Autodesk Inventor part; units mm, degrees
ref_plane "Work Plane3" through (0, 1.2, 0) normal (0, 1, 0) x (1, 0, 0)
ref_plane "YZ Plane" through (0, 0, 0) normal (1, 0, 0) x (0, 1, 0)
ref_plane "XZ Plane" through (0, 0, 0) normal (0, 1, 0) x (-1, 0, 0)
sketch "Sketch1" plane through (0, 0, 0) normal (0, 1, 0) x (-1, 0, 0)
  circle A0 centre (0, 0) radius 1.1
  arc A1 (3.1, 0) -> (-3.1, 0) centre (0, 0) ccw
  circle A2 centre (0, -58) radius 1.1
  arc A3 (-3.1, -58) -> (3.1, -58) centre (0, -58) ccw
  line L0 (3.1, -58) -> (3.1, -54.5)
  line L1 (-3.1, -58) -> (-3.1, -54.5)
  line L2 (3.1, -54.5) -> (-3.1, -54.5)
  line L3 (3.1, -3.5) -> (-3.1, -3.5)
  line L4 (-3.1, -3.5) -> (-3.1, 0)
  line L5 (3.1, 0) -> (3.1, -3.5)
  line L6 (3.1, -55.5) -> (-3.1, -55.5)
  line L7 (3.1, -2.5) -> (-3.1, -2.5)
  line L8 (-0.1, -2.5) -> (-0.1, -3.5)
  dimension "d0" = 2.2
  dimension "d1" = 2
  dimension "d2" = 2.2
  dimension "d3" = 2
  dimension "d4" = 58
  dimension "d5" = 3.5
  dimension "d6" = 3.5
  dimension "d7" = 1
  dimension "d8" = 1
  dimension "d17" = 0.1
extrude "Extrusion1" add sketch "Sketch1" along normal blind 2 contours L1 L6 L0 A3
extrude "Extrusion5" add sketch "Sketch1" along normal blind 1 contours L5 L7 L4 A1 | L5 L3 L8 L7
extrude "Extrusion2" add sketch "Sketch1" along normal blind 16.6 contours L7 L8 L3 L4 | L1 L2 L0 L6
sketch "Sketch2" plane through (0, 16.6, 0) normal (0, 1, 0) x (1, 0, 0)
  line L0 (-3.1, 2.5) -> (-3.1, 0) construction
  line L1 (3.1, 55.5) -> (3.1, 58) construction
  line L2 (-3.1, 2.5) -> (3.1, 2.5)
  line L3 (3.1, 2.5) -> (3.1, 55.5)
  line L4 (3.1, 55.5) -> (-3.1, 55.5)
  line L5 (-3.1, 55.5) -> (-3.1, 2.5)
  line L6 (3.1, 3.5) -> (0.1, 3.5) construction
  line L7 (-3.1, 54.5) -> (3.1, 54.5) construction
  line L8 (-1.7, 3.5) -> (1.7, 3.5)
  line L9 (1.7, 3.5) -> (1.7, 54.5)
  line L10 (1.7, 54.5) -> (-1.7, 54.5)
  line L11 (-1.7, 54.5) -> (-1.7, 3.5)
  line L12 (3.1, 3.5) -> (-3.1, 3.5)
  line L13 (-0.1, 3.5) -> (-0.1, 2.5)
  line L14 (0.1, 3.5) -> (0.1, 2.5)
  point P0 (0, 0)
  point P1 (0, 3.5)
  dimension "d13" = 1.4
  dimension "d14" = 1.4
  dimension "d37" = 0.2
  dimension "d38" = 0.1
extrude "Extrusion3" add sketch "Sketch2" along normal blind 2 contours L5 L12 L8 L13 L2 | L5 L4 L3 L12 L9 L10 L11 | L14 L8 L12 L3 L2
ref_plane "Work Plane3" through (0, 1.2, 0) normal (0, 1, 0) x (1, 0, 0)
sketch "Sketch4" plane through (0, 1.2, 0) normal (0, 1, 0) x (1, 0, 0)
  arc A0 (-3.1, 0) -> (3.1, 0) centre (0, 0) ccw
  circle A1 centre (0, 0) radius 1.1
  line L0 (-3.1, 3.5) -> (-3.1, 0) construction
  line L1 (3.1, 0) -> (3.1, 3.5) construction
  line L2 (3.1, 2.3) -> (3.1, 0)
  line L3 (3.1, 2.5) -> (0.1, 2.5) construction
  line L4 (-0.1, 2.3) -> (-0.1, 3.5)
  line L5 (-0.1, 3.5) -> (-3.1, 3.5)
  line L6 (3.1, 2.5) -> (0.1, 2.5)
  line L7 (-3.1, 2.5) -> (-0.1, 2.5)
  line L8 (-0.1, 2.3) -> (3.1, 2.3)
  line L9 (-3.1, 0) -> (-3.1, 3.5)
  dimension "d28" = 0.1
  dimension "d29" = 1
  dimension "d30" = 0.2
extrude "Extrusion6" add sketch "Sketch4" along normal blind 1
extrude "Extrusion8" add sketch "Sketch4" along normal up to surface (15.4 mm away) contours L9 L5 L4 L7
equation "\"d0\" = bolt_thread_diameter + 2 * tol"
equation "\"d1\" = thickness"
equation "\"d2\" = bolt_thread_diameter + 2 * tol"
equation "\"d3\" = thickness"
equation "\"d5\" = hole_pin_separation - tol"
equation "\"d6\" = hole_pin_separation - tol"
equation "\"d7\" = minor_thickness"
equation "\"d8\" = minor_thickness"
equation "\"d9\" = thickness"
equation "\"d24\" = 0.5 * thickness"
equation "\"d11\" = wire_height + pin_base_height + tol"
equation "\"d13\" = overhang"
equation "\"d14\" = overhang"
equation "\"d37\" = 2 * tol"
equation "\"d15\" = thickness"
equation "\"d29\" = minor_thickness"
equation "\"d30\" = 2 * tol"
equation "\"d31\" = 0.5 * thickness"
equation "\"d35\" = 0.5 * thickness"
equation "\"wire_height\" = 14"
equation "\"hole_separation\" = 58"
equation "\"pin_base_height\" = 2.5"
equation "\"hole_pin_separation\" = 3.6"
equation "\"minor_thickness\" = 1"
equation "\"overhang\" = 1.4"
equation "\"d26\" = 2 * tol"
properties part number "WIRE_HOUSING" material "PC/ABS Plastic"
Verification items for the finished model (mm, model axes). A direction names the side the tool comes from. Round coordinates to 2 decimals unless told otherwise and drop trailing zeros. Order: outer loops, then holes, each group sorted by start corner. A loop starts at its lowest first (then second) coordinate and runs counter-clockwise, first axis right, second up. Notation, with made-up numbers: (43, -32) -> (90, -32) arc R11 ccw to (90, -14) -> close; hole circle Ø11 at (54, -38.75). An arc over 180 degrees is marked (long way). Put each result on its own line as item: value.
1) Section check B-B (z = -37). Record the cut outline in (x, y).
Final values:
outline: (-3.1, 16.6) -> (-1.7, 16.6) -> (-1.7, 18.6) -> (-3.1, 18.6) -> close; (1.7, 16.6) -> (3.1, 16.6) -> (3.1, 18.6) -> (1.7, 18.6) -> close
2) Set-up check for faces 4 (the flat face through (0, 10, -55.5)), 5 (the flat face through (2, 16.6, -29)), 6 (the flat face through (1.7, 18, -29)): record each of +Z, -Z, +X, -X, +Y, -Y from which the full face is reachable in a straight line by a thin tool's end or side.
Final values:
face 4: -Z, +X, -X, +Y
face 5: +X, -X, -Y
face 6: +Y, -Y
3) Depth check by flat-ended pin: pin 1 (3 mm diameter, centred on x = -2, z = -18, fed in from -Y); pin 2 (1.8 mm diameter, centred on x = 0, z = -58, fed in from -Y); pin 3 (1.9 mm diameter, centred on x = -1.5, z = 1, fed in from +Y); pin 4 (3 mm diameter, centred on x = -1, z = 1, fed in from -Y). Enter the tip coordinate at first touch or a pass-through.
Final values:
pin 1: stops at y = 16.6
pin 2: passes through
pin 3: stops at y = 2.2
pin 4: stops at y = 0
4) Material ranges on line 1 (Z direction, x = 0, y = 0.5); line 2 (Z direction, x = 0, y = 1.75); line 3 (X direction, y = 1.7, z = 0), recorded low to high.
Final values:
line 1: z = -61.1 to -59.1, -56.9 to -54.5, -3.5 to -1.1, 1.1 to 3.1
line 2: z = -61.1 to -59.1, -56.9 to -54.5, -2.3 to -1.1, 1.1 to 3.1
line 3: x = -3.1 to -1.1, 1.1 to 3.1
5) Mould release check, pull along X, two halves, no side actions. Record for faces 1 (the flat face through (-3.1, 17, -29)), 2 (the flat face through (-2, 10, -2.5)), 3 (the cylindrical face through (-1.05, 0.49, -0.33)): +X half, -X half, draft (parallel to the pull), parting line (faces both ways), or undercut.
Final values:
face 1: -X half
face 2: draft
face 3: undercut
6) Section check A-A (y = 12.25). Record the cut outline in (x, z).
Final values:
outline: (-3.1, -55.5) -> (3.1, -55.5) -> (3.1, -54.5) -> (-3.1, -54.5) -> close; (-3.1, -3.5) -> (-0.1, -3.5) -> (-0.1, -2.5) -> (-3.1, -2.5) -> close; (0.1, -3.5) -> (3.1, -3.5) -> (3.1, -2.5) -> (0.1, -2.5) -> close
7) Section check C-C (x = 2.5). Record the cut outline in (y, z).
Final values:
outline: (0, -59.83) -> (2, -59.83) -> (2, -55.5) -> (18.6, -55.5) -> (18.6, -2.5) -> (1, -2.5) -> (1, 1.83) -> (0, 1.83) -> (0, -3.5) -> (16.6, -3.5) -> (16.6, -54.5) -> (0, -54.5) -> close; (1.2, -2.3) -> (2.2, -2.3) -> (2.2, 1.83) -> (1.2, 1.83) -> close
